Part model, mm, in its own coordinate system. Face numbers are marked on the shaded views. Give positions to 0.01 mm unless a question says otherwise; leave off trailing zeros. Order: outer loops, then holes, each group sorted by start corner. A loop starts at its lowest first (then second) coordinate and runs counter-clockwise, first axis right, second up.
1. Drop flat-ended pins along their axis: pin 1 Ø1.8 at (y, z) = (7, 0) entering from +X; pin 2 Ø10 at (x, y) = (27.5, -1) entering from +Z; pin 3 Ø6 at (x, y) = (47, 4) entering from -Z; pin 4 Ø8 at (x, y) = (15, -5.5) entering from -Z. Give the stop position or say it passes through.
2. Mould opens along X. For the marked faces 1, 2 and 3 say: +X half, -X half, draft (parallel to the pull), parting line (faces both ways), or undercut.
3. Slice it at C-C on z = -7. List the corners of the cut face in (x, y), and give its area (3 significant figures).
4. Slice it at B-B on z = 0.75. List the corners of the cut face in (x, y).
5. Slice it at A-A on y = 0. List the corners of the cut face in (x, z).
6. Probe line 1 (Y direction, x = 53.9, z = 0); line 2 (X direction, y = -7.5, z = -5.75); line 3 (Y direction, x = 54.6, z = 7). List the from-to ranges inside material, lowest first.
from build123d import *

# Parameters (mm, degrees)
CROQUIS1_R              = 10
SALIENTE_EXTRUIR1_DEPTH = 2.7
CROQUIS2_R              = 5
SALIENTE_EXTRUIR2_DEPTH = 50
CROQUIS3_R              = 10
SALIENTE_EXTRUIR3_DEPTH = 2.7
CROQUIS5_R              = 1.5
CORTAR_EXTRUIR1_DEPTH   = 60


with BuildPart() as part:
    # Croquis1 → Saliente-Extruir1 (new body)
    with BuildSketch(Plane(origin=(0, 0, 0), x_dir=(0, 0, -1), z_dir=(1, 0, 0))):
        with Locations(Location((0, 0, 0), (0, 0, 180))):
            Circle(CROQUIS1_R)
    extrude(amount=SALIENTE_EXTRUIR1_DEPTH)

    # Croquis2 → Saliente-Extruir2 (add)
    with BuildSketch(Plane(origin=(2.7, 0, 0), x_dir=(0, 0, -1), z_dir=(1, 0, 0))):
        Circle(CROQUIS2_R)
    extrude(amount=SALIENTE_EXTRUIR2_DEPTH)

    # Croquis3 → Saliente-Extruir3 (add)
    with BuildSketch(Plane(origin=(52.7, 0, 0), x_dir=(0, 0, -1), z_dir=(1, 0, 0))):
        with Locations(Location((0, 0, 0), (0, 0, 180))):
            Circle(CROQUIS3_R)
    extrude(amount=SALIENTE_EXTRUIR3_DEPTH)

    # Croquis5 → Cortar-Extruir1 (cut)
    with BuildSketch(Plane(origin=(55.4, 0, 0), x_dir=(0, 0, -1), z_dir=(1, 0, 0))):
        with Locations((0, 7)):
            Circle(CROQUIS5_R)
        with Locations((7, 0)):
            Circle(CROQUIS5_R)
        with Locations((0, -7)):
            Circle(CROQUIS5_R)
        with Locations((-7, 0)):
            Circle(CROQUIS5_R)
    extrude(amount=-CORTAR_EXTRUIR1_DEPTH, mode=Mode.SUBTRACT)


solid = part.part
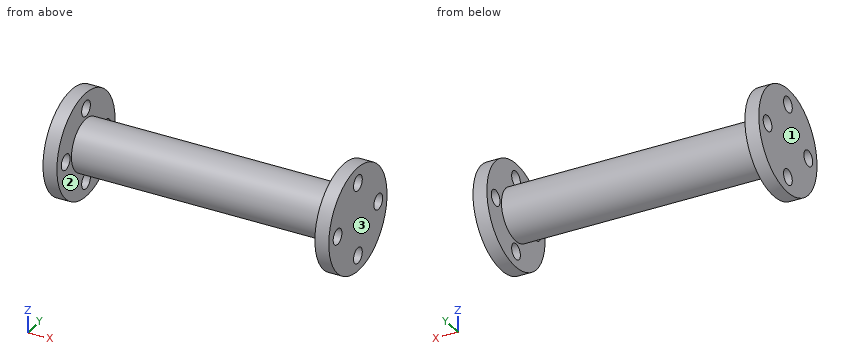
Data:
1. pin 1: passes through
1. pin 2: stops at z = 5
1. pin 3: stops at z = -4.9
1. pin 4: stops at z = -4.77
2. face 1: -X half
2. face 2: undercut
2. face 3: +X half
3. outline: (0, -7.14) - (2.7, -7.14) - (2.7, -1.5) - (0, -1.5) - close; (0, 1.5) - (2.7, 1.5) - (2.7, 7.14) - (0, 7.14) - close; (52.7, -7.14) - (55.4, -7.14) - (55.4, -1.5) - (52.7, -1.5) - close; (52.7, 1.5) - (55.4, 1.5) - (55.4, 7.14) - (52.7, 7.14) - close
3. area: 60.9 mm2
4. outline: (0, -9.97) - (2.7, -9.97) - (2.7, -8.3) - (0, -8.3) - close; (0, -5.7) - (2.7, -5.7) - (2.7, -4.94) - (52.7, -4.94) - (52.7, -5.7) - (55.4, -5.7) - (55.4, 5.7) - (52.7, 5.7) - (52.7, 4.94) - (2.7, 4.94) - (2.7, 5.7) - (0, 5.7) - close; (0, 8.3) - (2.7, 8.3) - (2.7, 9.97) - (0, 9.97) - close; (52.7, -9.97) - (55.4, -9.97) - (55.4, -8.3) - (52.7, -8.3) - close; (52.7, 8.3) - (55.4, 8.3) - (55.4, 9.97) - (52.7, 9.97) - close
5. outline: (0, -10) - (2.7, -10) - (2.7, -8.5) - (0, -8.5) - close; (0, -5.5) - (2.7, -5.5) - (2.7, -5) - (52.7, -5) - (52.7, -5.5) - (55.4, -5.5) - (55.4, 5.5) - (52.7, 5.5) - (52.7, 5) - (2.7, 5) - (2.7, 5.5) - (0, 5.5) - close; (0, 8.5) - (2.7, 8.5) - (2.7, 10) - (0, 10) - close; (52.7, -10) - (55.4, -10) - (55.4, -8.5) - (52.7, -8.5) - close; (52.7, 8.5) - (55.4, 8.5) - (55.4, 10) - (52.7, 10) - close
6. line 1: y = -10 to -8.5, -5.5 to 5.5, 8.5 to 10
6. line 2: x = 0 to 2.7, 52.7 to 55.4
6. line 3: y = -7.14 to -1.5, 1.5 to 7.14
